Work out the finished part from the listing and answer in its coordinate system (mm). Face numbers are marked on the shaded views. A direction names the side the tool comes from. Round coordinates to 2 decimals unless told otherwise and drop trailing zeros. Loops run counter-clockwise (first coordinate to the right, second up) from the corner with the lowest first, then second, coordinate; pieces in that order, holes last. Notation, with made-up numbers: (-16.5, 32.5) - (-12.5, 32.5) arc R16 ccw to (-12.5, 37.5) - close; hole circle Ø3 at (-20, 89). An arc over 180 degrees is marked (long way). Answer as CSV lines item,"result". Start each with the question number.
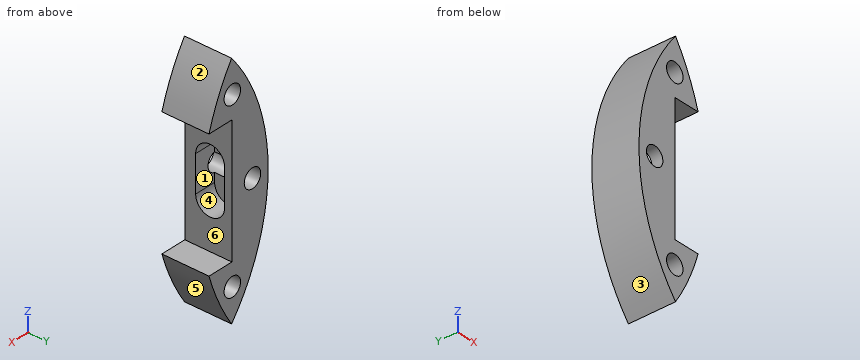
```python
from build123d import *

# Parameters (mm, degrees)
SKETCH_1_R          = 2.6
EXTRUDE_1_DEPTH     = 13
CUT_EXTRUDE_1_DEPTH = 6


with BuildPart() as part:
    # 草图1 → 凸台-拉伸1 (new body)
    with BuildSketch(Plane(origin=(0, 0, 0), x_dir=(1, 0, 0), z_dir=(0, 1, 0))):
        with BuildLine():
            Line((-33.760275315, -17.55), (-41, -17.55))
            Line((-41, -17.55), (-41, 17.55))
            Line((-41, 17.55), (-33.760275315, 17.55))
            ThreePointArc((-33.760275315, 17.55), (-36.796000438, 25.438985546), (-40.910253672, 32.823065739))
            ThreePointArc((-40.910253672, 32.823065739), (-52.45, 0), (-40.910253672, -32.823065739))
            ThreePointArc((-40.910253672, -32.823065739), (-36.796000438, -25.438985546), (-33.760275315, -17.55))
        make_face()
        with Locations(Location((-41.13620668, -23.75, 0), (0, 0, 90))):
            Circle(SKETCH_1_R, mode=Mode.SUBTRACT)
        with Locations(Location((-41.13620668, 23.75, 0), (0, 0, 90))):
            Circle(SKETCH_1_R, mode=Mode.SUBTRACT)
        with Locations(Location((-47.5, 0, 0), (0, 0, 90))):
            Circle(SKETCH_1_R, mode=Mode.SUBTRACT)
    extrude(amount=EXTRUDE_1_DEPTH)

    # 草图3 → 切除-拉伸1 (cut)
    with BuildSketch(Plane(origin=(-41, 0, 0), x_dir=(0, 0, -1), z_dir=(1, 0, 0))):
        with BuildLine():
            Line((-5, 11), (5, 11))
            ThreePointArc((5, 11), (9, 7), (5, 3))
            Line((5, 3), (-5, 3))
            ThreePointArc((-5, 3), (-9, 7), (-5, 11))
        make_face()
    extrude(amount=-CUT_EXTRUDE_1_DEPTH, mode=Mode.SUBTRACT)


solid = part.part
```
Item 1: Flat-ended cylindrical pins translate along their axes: pin 1 Ø3 at (x, z) = (-44.5, -13.5) entering from -Y; pin 2 Ø4 at (x, y) = (-49, 4.5) entering from -Z; pin 3 Ø6 at (x, y) = (-36, 5) entering from -Z; pin 4 Ø1 at (x, y) = (-37.5, 8) entering from -Z. Find the tip coordinate at first contact, or state that the pin passes through.
Item 2: Find the intervals of material crossed by L1, parallel to Z at x = -42, y = 5; L2, parallel to Z at x = -43.5, y = 2.5; L3, parallel to Z at x = -43.25, y = 8, in increasing order.
Item 3: Section C-C, the plane x = -39.5 is taken. Give the vertices of the cut face in (y, z), and give its area (3 significant figures).
Item 4: Section A-A, the plane z = 0 is taken. Give the vertices of the cut face in (x, y).
Item 5: Section B-B, the plane y = 9 is taken. Give the vertices of the cut face in (x, z).
Item 6: Determine the mould class of the marked faces 1, 2 and 3 for opening direction Z: pulls with the +Z half, pulls with the -Z half, needs draft (parallel to the pull), parting line crosses it, or undercut.
Item 7: Section D-D, the plane y = 11.75 is taken. Give the vertices of the cut face in (x, z).
Item 8: Which of the six approach directions +Z, -Z, +X, -X, +Y, -Y give full straight-line access (tool end or side, diameter ignored) to the marked faces 4, 5 and 6?
Answer:
1,pin 1,"stops at y = 0"
1,pin 2,"stops at z = -23.28"
1,pin 3,"stops at z = -29.7"
1,pin 4,"stops at z = -27.87"
2,L1,"z = -31.42 to -26.2, -21.3 to -8.46, 8.46 to 21.3, 26.2 to 31.42"
2,L2,"z = -29.3 to -24.83, -22.67 to 22.67, 24.83 to 29.3"
2,L3,"z = -29.67 to -25.26, -22.24 to -8.87, 8.87 to 22.24, 25.26 to 29.67"
3,outline,"(0, -30.56) - (13, -30.56) - (13, -25.77) - (0, -25.77) - close; (0, -21.73) - (13, -21.73) - (13, -17.55) - (0, -17.55) - close; (0, 17.55) - (13, 17.55) - (13, 21.73) - (0, 21.73) - close; (0, 25.77) - (13, 25.77) - (13, 30.56) - (0, 30.56) - close"
3,area,"233 mm²"
4,outline,"(-52.45, 0) - (-50.1, 0) - (-50.1, 13) - (-52.45, 13) - close; (-44.9, 0) - (-41, 0) - (-41, 3) - (-44.9, 3) - close; (-44.9, 11) - (-41, 11) - (-41, 13) - (-44.9, 13) - close"
5,outline,"(-47, -8.46) - (-47, -2.55) arc R2.6 cw (long way) to (-47, 2.55) - (-47, 8.46) - (-41, 8.46) - (-41, 17.55) - (-33.76, 17.55) arc R60 ccw to (-40.91, 32.82) arc R52.45 ccw to (-40.91, -32.82) arc R60 ccw to (-33.76, -17.55) - (-41, -17.55) - (-41, -8.46) - close; hole circle Ø5.2 at (-41.14, -23.75); hole circle Ø5.2 at (-41.14, 23.75)"
6,face 1,"undercut"
6,face 2,"pulls with the +Z half"
6,face 3,"parting line crosses it"
7,outline,"(-41, -17.55) - (-41, 17.55) - (-33.76, 17.55) arc R60 ccw to (-40.91, 32.82) arc R52.45 ccw to (-40.91, -32.82) arc R60 ccw to (-33.76, -17.55) - close; hole circle Ø5.2 at (-47.5, 0); hole circle Ø5.2 at (-41.14, -23.75); hole circle Ø5.2 at (-41.14, 23.75)"
8,face 4,"+X"
8,face 5,"-Z, +X, +Y, -Y"
8,face 6,"+X, +Y, -Y"
